Geometry check sheet. Reference: the model listing, model coordinates, mm. Give positions to 0.01 mm unless a question says otherwise; leave off trailing zeros. Order: outer loops, then holes, each group sorted by start corner. A loop starts at its lowest first (then second) coordinate and runs counter-clockwise, first axis right, second up. Notation, with made-up numbers: M 46,-2.75 L 93,-2.75 A21 cw 93,32.25 Z; hole C 89,-13.75 d4. An arc over 180 degrees is marked long. Use CSV: the item, a comma, the result in double quotes. Start each with the question number.
from build123d import *


# Not quite as in the source:
# - a feature names something its author has since deleted; it is built from what else it names


with BuildPart() as f1:
    # F0 (on Front) → F1 (revolve)
    with BuildSketch(Plane.XZ):
        with BuildLine():
            Line((0, 0), (0, -38.1))
            ThreePointArc((0, -38.1), (36.8901663726, -9.525), (18.4450831863, 33.3375))
            ThreePointArc((18.4450831863, 33.3375), (24.8680463142, 55.9710997394), (9.9547263147, 74.168))
            ThreePointArc((9.9547263147, 74.168), (17.7294771599, 90.2394176477), (7.6284402255, 104.9603642464))
            ThreePointArc((7.6284402255, 104.9603642464), (12.0633962281, 108.7560954443), (17.78, 109.9379801202))
            Line((17.78, 109.9379801202), (17.78, 117.5579801202))
            Line((17.78, 117.5579801202), (10.1936982811, 117.5579801202))
            Line((10.1936982811, 117.5579801202), (18.0881139505, 143.3620005846))
            Line((18.0881139505, 143.3620005846), (0, 143.3620005846))
            Line((0, 143.3620005846), (0, 0))
        make_face()
    revolve(axis=Axis((0, 0, 71.6810002923), (0, 0, -1)))


solid = f1.part
(1) Draft check along Z on faces 1 (the face through (0, 0, 143.362)), 2 (the face through (-3.85, 17.36, 113.8)), 3 (the face through (8, 8, 117.558)). Enter one of: +Z half, -Z half, draft (parallel to the pull), parting line (faces both ways), or undercut.
(2) Sectioned sample at A-A on y = 0. Record the cut outline in (x, z).
(3) Sectioned sample at D-D on y = -21.5. Record the cut outline in (x, z), then the cut area to 3 significant figures.
(4) Thickness scan on line 1 (Z direction, x = -20, y = -4.5); line 2 (Z direction, x = 5, y = 19); line 3 (Y direction, x = -22, z = -9). Record the ranges inside material, lowest first.
(5) Go/stop test with flat-tipped pins: P1, Ø8, axis at x = -11, z = 48, coming from the -Y side; P2, Ø1.5, axis at x = 17, y = 0.5, coming from the -Z side; P3, Ø6, axis at y = 19.5, z = 39.5, coming from the +X side. Record where each tip stops, or that it passes through.
(6) Sectioned sample at C-C on z = -4. Record the cut outline in (x, y), then the cut area to 3 significant figures.
Responses:
1,face 1,"+Z half"
1,face 2,"undercut"
1,face 3,"undercut"
2,outline,"M -18.45,33.34 A38.1 ccw long 18.45,33.34 A25.4 ccw 9.95,74.17 A17.78 ccw 7.63,104.96 A11.71 cw 17.78,109.94 L 17.78,117.56 L 10.19,117.56 L 18.09,143.36 L -18.09,143.36 L -10.19,117.56 L -17.78,117.56 L -17.78,109.94 A11.71 cw -7.63,104.96 A17.78 ccw -9.95,74.17 A25.4 ccw Z"
3,outline,"C 0,0 d62.91; C 0,50.8 d27.05"
3,area,"3,680 mm2"
4,line 1,"-32.11 to 32.11, 35.8 to 65.8"
4,line 2,"-32.64 to 32.64, 34.7 to 66.9"
4,line 3,"-29.78 to 29.78"
5,P1,"y = -24.31"
5,P2,"z = -34.46"
5,P3,"x = 16.23"
6,outline,"C 0,0 d75.78"
6,area,"4,510 mm2"
